Here's the drawing with two shaded views (mm, measured from the low corner). I have some questions. A direction names the side the tool comes from. Round coordinates to 2 decimals unless told otherwise and drop trailing zeros. Loops run counter-clockwise (first coordinate to the right, second up) from the corner with the lowest first, then second, coordinate; pieces in that order, holes last.
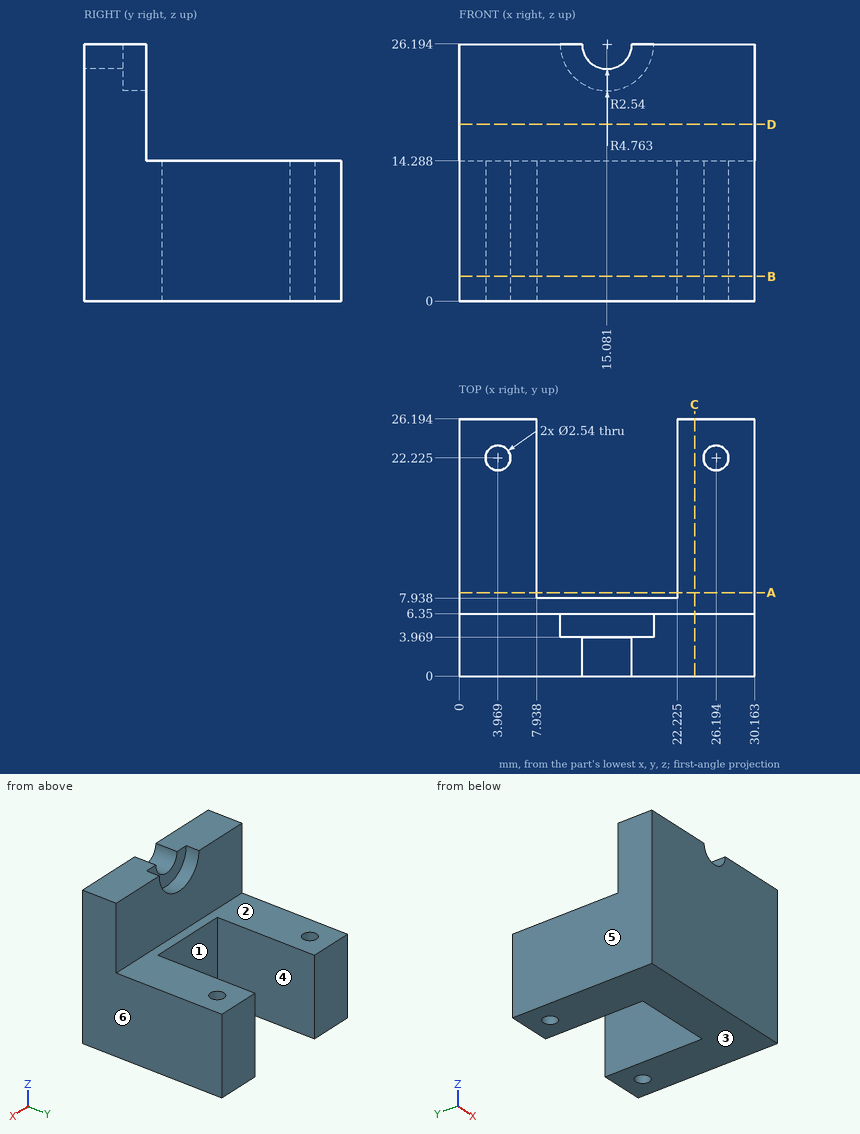
(1) If we section it at C-C, the plane x = 24: List the corners of the cut face in (y, z) for me, then the cut area to 3 significant figures.
Worked answers:
outline: (0, 0) - (26.19, 0) - (26.19, 14.29) - (6.35, 14.29) - (6.35, 26.19) - (0, 26.19) - close
area: 450 mm2
(2) For the marked faces 1, 2 and 3, which set-ups out of +Z, -Z, +X, -X, +Y, -Y let a thin tool reach every point of the face, with its end or its side?
Worked answers:
face 1: +Z, -Z, +Y
face 2: +Z, +X, -X, +Y
face 3: -Z, +X, -X, +Y, -Y
(3) Will these pins go through, and if not, where does the flat tip stop? P1, Ø2.5, axis at x = 13, z = 24, coming from the +Y side; P2, Ø3.5, axis at x = 11.5, z = 18.5, coming from the +Y side; P3, Ø4.5, axis at x = 16, z = 9.5, coming from the +Y side.
Worked answers:
P1: stops at y = 3.97
P2: stops at y = 6.35
P3: stops at y = 7.94
(4) If we section it at A-A, the plane y = 8.5: List the corners of the cut face in (x, z) for me (1 decimal).
Worked answers:
outline: (0, 0) - (7.9, 0) - (7.9, 14.3) - (0, 14.3) - close; (22.2, 0) - (30.2, 0) - (30.2, 14.3) - (22.2, 14.3) - close
(5) If we section it at D-D, the plane z = 18: List the corners of the cut face in (x, y) for me.
Worked answers:
outline: (0, 0) - (30.16, 0) - (30.16, 6.35) - (0, 6.35) - close
(6) If we section it at B-B, the plane z = 2.5: List the corners of the cut face in (x, y) for me (1 decimal), then the cut area to 3 significant figures.
Worked answers:
outline: (0, 0) - (30.2, 0) - (30.2, 26.2) - (22.2, 26.2) - (22.2, 7.9) - (7.9, 7.9) - (7.9, 26.2) - (0, 26.2) - close; hole circle Ø2.5 at (4, 22.2); hole circle Ø2.5 at (26.2, 22.2)
area: 519 mm2
(7) If we mould it in two halves opening along X, with no side actions, what happens to the marked faces 4, 5 and 6? For each: released by +X, released by -X, zero draft, split by the parting line, or undercut.
Worked answers:
face 4: undercut
face 5: released by -X
face 6: released by +X
(8) If I drill on line 1 (X direction, y = 11, z = 9.25) (1 decimal); line 2 (Y direction, x = 8.5, z = 11.5); line 3 (Y direction, x = 2.5, z = 20.5), over which ranges is the centre line in solid material (lowest first)?
Worked answers:
line 1: x = 0 to 7.9, 22.2 to 30.2
line 2: y = 0 to 7.94
line 3: y = 0 to 6.35
